Build history of the part. All positions in model axes, mm. A direction names the side the tool comes from. Give positions to 0.01 mm unless a question says otherwise; leave off trailing zeros. Write each loop counter-clockwise with the first axis right and the second up, starting at its lowest first coordinate (ties: lowest second). Pieces come first, ordered by that corner, then holes. Notation, with made-up numbers: (16.5, 89.5) -> (57.5, 89.5) arc R12 cw to (57.5, 105.5) -> close; hole circle Ø9 at (66.25, 67). An arc over 180 degrees is marked (long way). Put each result on its own line as item: value. Start each with the question number.
Item 1: Flat gauge pins, fed straight in: pin 1 Ø11 at (y, z) = (4.5, -134) entering from +X; pin 2 Ø4 at (y, z) = (19.5, -18) entering from +X; pin 3 Ø11 at (x, y) = (-65.5, 43) entering from -Z. Where does each tip first touch, or does it go through?
Item 2: Slice it at D-D, the plane z = -33.5. List the corners of the cut face in (x, y), plus the area to 3 significant figures.
Item 3: Drill centre lines: line 1 along X through (y, z) = (58.2, -20); line 2 along Y through (x, z) = (-37, -37.5); line 3 along X through (y, z) = (50, -42). Where is each one in solid material? Low to high.
Item 4: Tool access for faces 5 (the flat face through (-61, 50, -112)), 6 (the flat face through (0, 57, -20)), 7 (the flat face through (-25, 5, -24)), 8 (the flat face through (-39.72, 54.93, -126.523)): list every direction of +Z, -Z, +X, -X, +Y, -Y with a clear straight run to the whole face (end or side of a thin tool).
Item 5: Two-plate mould, pull along Y, no slides. Class faces 1 (the flat face through (-65, 42, -70)), 2 (the flat face through (-42, 0, -38)), 3 (the cylindrical face through (-15.12, 57.46, -21.08)), 4 (the flat face through (-50, 30, -20)): pulls with the +Y half, pulls with the -Y half, needs draft (parallel to the pull), parting line crosses it, or undercut.
Item 6: Slice it at C-C, the plane y = 28. List the corners of the cut face in (x, z), plus the area to 3 significant figures.
Item 7: Slice it at A-A, the plane z = -101. List the corners of the cut face in (x, y), plus the area to 3 significant figures.
Item 8: Slice it at B-B, the plane x = -57. List the corners of the cut face in (y, z), plus the area to 3 significant figures.
Autodesk Inventor part; units mm, degrees
ref_plane "YZ Plane" through (0, 0, 0) normal (1, 0, 0) x (0, 1, 0)
ref_plane "XZ Plane" through (0, 0, 0) normal (0, 1, 0) x (-1, 0, 0)
ref_plane "XY Plane" through (0, 0, 0) normal (0, 0, 1) x (1, 0, 0)
sketch "스케치1" plane through (0, 0, 0) normal (0, 1, 0) x (-1, 0, 0)
  line L0 (0, 0) -> (70, 0)
  line L1 (70, 0) -> (70, -140)
  line L2 (70, -140) -> (20, -140)
  line L3 (20, -140) -> (20, -130)
  line L4 (20, -130) -> (60, -122.9469)
  line L5 (60, -122.9469) -> (60, -40)
  line L6 (60, -40) -> (0, -40)
  line L7 (0, -40) -> (0, 0)
  dimension "d0" = 60
  dimension "d1" = 40
  dimension "d2" = 140
  dimension "d3" = 50
  dimension "d4" = 100
  dimension "d5" = 10
  dimension "d6" = 70
extrude "돌출1" add sketch "스케치1" along normal blind 60
sketch "스케치2" plane through (0, 0, 0) normal (1, 0, 0) x (0, 0, -1)
  line L0 (40, 0) -> (0, 0)
  line L1 (40, 0) -> (40, 60)
  line L2 (0, 60) -> (40, 60)
  line L3 (0, 0) -> (0, 60)
  line L4 (40, 0) -> (40, 60)
  line L5 (0, 5) -> (40, 5)
  line L6 (40, 5) -> (40, 55)
  line L7 (40, 55) -> (0, 55)
  line L8 (0, 55) -> (0, 5)
  dimension "d9" = 5
  dimension "d10" = 5
extrude "돌출2" cut sketch "스케치2" against normal blind 50 contours L5 L3 L7 L1
sketch "스케치3" plane through (-20, 0, -130) normal (1, 0, 0) x (0, 0, -1)
  line L0 (10, 0) -> (0, 0)
  line L1 (10, 0) -> (10, 60)
  line L2 (0, 60) -> (10, 60)
  line L3 (0, 0) -> (0, 60)
  line L4 (10, 35) -> (-60, 35)
  line L5 (-60, 35) -> (-60, 50)
  line L6 (-60, 50) -> (10, 50)
  line L7 (10, 50) -> (10, 35)
  line L8 (10, 0) -> (10, 60)
  line L9 (10, 10) -> (-60, 10)
  line L10 (-60, 10) -> (-60, 25)
  line L11 (-60, 25) -> (10, 25)
  line L12 (10, 25) -> (10, 10)
  line L13 (-90, 60) -> (-7.0531, 60)
  line L14 (-7.0531, 0) -> (-90, 0)
  point P0 (-130, 0)
  dimension "d13" = 70
  dimension "d14" = 15
  dimension "d15" = 70
  dimension "d16" = 15
  dimension "d17" = 10
  dimension "d18" = 10
extrude "돌출3" cut sketch "스케치3" against normal blind 50 contours L9 L3 L11 L1 | L9 L10 L11 L3 | L4 L3 L6 L1 | L4 L5 L6 L3
sketch "스케치4" plane through (0, 60, 0) normal (0, 1, 0) x (1, 0, 0)
  line L0 (-70, 0) -> (0, 0)
  line L1 (0, 0) -> (0, 40)
  point P0 (-20, 20)
  dimension "d21" = 20
  dimension "d22" = 20
hole "구멍1" at (-20, 60, -20) direction (0, -1, 0) diameter 10 end through all
properties part number "claw"
Values follow:
1. pin 1: x = -20
1. pin 2: x = -50
1. pin 3: z = -70
2. outline: (-70, 0) -> (0, 0) -> (0, 5) -> (-50, 5) -> (-50, 55) -> (0, 55) -> (0, 60) -> (-70, 60) -> close
2. area: 1,700 mm2
3. line 1: -70 to -25, -15 to 0
3. line 2: 0 to 5, 55 to 60
3. line 3: -70 to -60
4. face 5: -Z, +X, -X
4. face 6: +Z, -Z, +X, +Y, -Y
4. face 7: +Z, +X
4. face 8: +X, +Y, -Y
5. face 1: undercut
5. face 2: pulls with the -Y half
5. face 3: needs draft
5. face 4: undercut
6. outline: (-70, -140) -> (-20, -140) -> (-20, -130) -> (-60, -122.95) -> (-60, -40) -> (-50, -40) -> (-50, 0) -> (-70, 0) -> close
6. area: 2,340 mm2
7. outline: (-70, 0) -> (-60, 0) -> (-60, 10) -> (-70, 10) -> close; (-70, 25) -> (-60, 25) -> (-60, 35) -> (-70, 35) -> close; (-70, 50) -> (-60, 50) -> (-60, 60) -> (-70, 60) -> close
7. area: 300 mm2
8. outline: (0, -140) -> (10, -140) -> (10, -123.48) -> (0, -123.48) -> close; (0, -40) -> (60, -40) -> (60, 0) -> (0, 0) -> close; (25, -140) -> (35, -140) -> (35, -123.48) -> (25, -123.48) -> close; (50, -140) -> (60, -140) -> (60, -123.48) -> (50, -123.48) -> close
8. area: 2,900 mm2
